Could you check a few things on this model? Use its own coordinates, in mm. Face numbers are marked on the shaded views. A direction names the side the tool comes from. Give positions to 0.01 mm unless a question says otherwise; leave off trailing zeros. Loops run counter-clockwise (first coordinate to the right, second up) from the corner with the lowest first, then second, coordinate; pieces in that order, holes last. Notation, with made-up numbers: (84.5, 22.25) - (94.5, 22.25) arc R24 cw to (94.5, 52.25) - close; hole circle Ø8 at (-19.5, 61.5). An arc over 180 degrees is marked (long way). One line per item, written item: value. Start each with the question number.
Q1. If I drill on line 1 (Z direction, x = -14, y = -12); line 2 (Y direction, x = -11, z = 5.5) (3 decimals); line 3 (Y direction, x = -13.5, z = 6.5), over which ranges is the centre line in solid material (lowest first)? Write a range as from..to.
Q2. I want a section at B-B (z = 2.75). Please give me the cut outline in (x, y), then the cut area to 3 significant figures.
Q3. I'm going to push flat-ended pins straight in: P1, Ø5, axis at y = 15, z = 13, coming from the +X side; P2, Ø2, axis at y = 40, z = 17.5, coming from the +X side; P3, Ø2.5, axis at x = 20, y = 0, coming from the +Z side; P4, Ø4.5, axis at x = -20, y = 0, coming from the +Z side. Where does each tip first touch, or does it pass through?
Q4. If we mould it in two halves opening along Y, with no side actions, what happens to the marked faces 5, 6 and 7? For each: released by +Y, released by -Y, zero draft, split by the parting line, or undercut.
Q5. I want a section at C-C (x = -20). Please give me the cut outline in (y, z), then the cut area to 3 significant figures.
Q6. For the marked faces 1, 2, 3 and 4, which set-ups out of +Z, -Z, +X, -X, +Y, -Y let a thin tool reach every point of the face, with its end or its side?
Q7. I want a section at D-D (y = -7). Please give me the cut outline in (x, z), then the cut area to 3 significant figures.
Q8. I want a section at A-A (z = 13). Count the separate pieces of the cut face and the enclosed holes in it, then the cut area to 3 significant figures.
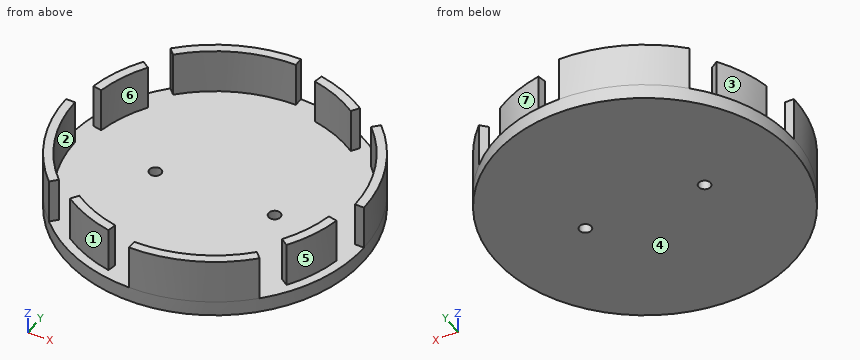
```python
from build123d import *
from build123d.topology import SkipClean

# Parameters (mm, degrees)
SKETCH_1_R      = 50
SKETCH_1_R_2    = 2
EXTRUDE_1_DEPTH = 5
EXTRUDE_2_DEPTH = 15
EXTRUDE_3_DEPTH = 15
EXTRUDE_4_DEPTH = 15


with BuildPart() as part:
    # 草图1 → 凸台-拉伸1 (new body)
    with BuildSketch(Plane.XY):
        Circle(SKETCH_1_R)
        with Locations((-20, 0)):
            Circle(SKETCH_1_R_2, mode=Mode.SUBTRACT)
        with Locations((20, 0)):
            Circle(SKETCH_1_R_2, mode=Mode.SUBTRACT)
    extrude(amount=EXTRUDE_1_DEPTH)

    # 草图2 → 凸台-拉伸2 (add)
    with SkipClean():  # the faces are left unmerged after this step: merging them gives an invalid solid
        with BuildSketch(Plane.XY.offset(5)):
            with BuildLine():
                Line((0, 50), (0, 47))
                ThreePointArc((0, 47), (-17.986121321, 43.422338028), (-33.234018716, 33.234018716))
                Line((-33.234018716, 33.234018716), (-35.355339059, 35.355339059))
                ThreePointArc((-35.355339059, 35.355339059), (-19.134171618, 46.193976626), (0, 50))
            make_face()
        extrude(amount=EXTRUDE_2_DEPTH)

    # 草图5 → 凸台-拉伸3 (add)
    with SkipClean():  # the faces are left unmerged after this step: merging them gives an invalid solid
        with BuildSketch(Plane.XY.offset(5)):
            with BuildLine():
                Line((-35.355339059, 35.355339059), (-33.234018716, 33.234018716))
                ThreePointArc((-33.234018716, 33.234018716), (-17.986121321, 43.422338028), (0, 47))
                Line((0, 47), (0, 50))
                ThreePointArc((0, 50), (-19.134171618, 46.193976626), (-35.355339059, 35.355339059))
            make_face()
            with BuildLine():
                Line((-50, 0), (-47, 0))
                ThreePointArc((-47, 0), (-43.422338028, -17.986121321), (-33.234018716, -33.234018716))
                Line((-33.234018716, -33.234018716), (-35.355339059, -35.355339059))
                ThreePointArc((-35.355339059, -35.355339059), (-46.193976626, -19.134171618), (-50, 0))
            make_face()
            with BuildLine():
                Line((33.234018716, 33.234018716), (35.355339059, 35.355339059))
                ThreePointArc((35.355339059, 35.355339059), (46.193976626, 19.134171618), (50, 0))
                Line((50, 0), (47, 0))
                ThreePointArc((47, 0), (43.422338028, 17.986121321), (33.234018716, 33.234018716))
            make_face()
            with BuildLine():
                Line((0, -47), (0, -50))
                ThreePointArc((0, -50), (19.134171618, -46.193976626), (35.355339059, -35.355339059))
                Line((35.355339059, -35.355339059), (33.234018716, -33.234018716))
                ThreePointArc((33.234018716, -33.234018716), (17.986121321, -43.422338028), (0, -47))
            make_face()
        extrude(amount=EXTRUDE_3_DEPTH)

    # 草图6 → 凸台-拉伸4 (add)
    with SkipClean():  # the faces are left unmerged after this step: merging them gives an invalid solid
        with BuildSketch(Plane.XY.offset(5)):
            with BuildLine():
                Line((-39.079071778, 26.111800952), (-36.584662941, 24.445090253))
                ThreePointArc((-36.584662941, 24.445090253), (-40.65069943, 16.838071024), (-43.154552338, 8.583974169))
                Line((-43.154552338, 8.583974169), (-46.096908179, 9.169245135))
                ThreePointArc((-46.096908179, 9.169245135), (-43.422338028, 17.986121321), (-39.079071778, 26.111800952))
            make_face()
            with BuildLine():
                Line((9.169245135, 46.096908179), (8.583974169, 43.154552338))
                ThreePointArc((8.583974169, 43.154552338), (16.838071024, 40.65069943), (24.445090253, 36.584662941))
                Line((24.445090253, 36.584662941), (26.111800952, 39.079071778))
                ThreePointArc((26.111800952, 39.079071778), (17.986121321, 43.422338028), (9.169245135, 46.096908179))
            make_face()
            with BuildLine():
                Line((46.096908179, -9.169245135), (43.154552338, -8.583974169))
                ThreePointArc((43.154552338, -8.583974169), (40.65069943, -16.838071024), (36.584662941, -24.445090253))
                Line((36.584662941, -24.445090253), (39.079071778, -26.111800952))
                ThreePointArc((39.079071778, -26.111800952), (43.422338028, -17.986121321), (46.096908179, -9.169245135))
            make_face()
            with BuildLine():
                Line((-9.169245135, -46.096908179), (-8.583974169, -43.154552338))
                ThreePointArc((-8.583974169, -43.154552338), (-16.838071024, -40.65069943), (-24.445090253, -36.584662941))
                Line((-24.445090253, -36.584662941), (-26.111800952, -39.079071778))
                ThreePointArc((-26.111800952, -39.079071778), (-17.986121321, -43.422338028), (-9.169245135, -46.096908179))
            make_face()
        extrude(amount=EXTRUDE_4_DEPTH)


solid = part.part
```
Worked answers:
1. line 1: z = 0..5
1. line 2: y = -45.695..-42.603, 45.695..48.775
1. line 3: y = -45.02..-41.88, 45.02..48.14
2. outline: circle Ø100 at (0, 0); hole circle Ø4 at (-20, 0); hole circle Ø4 at (20, 0)
2. area: 7,830 mm²
3. P1: stops at x = 48.41
3. P2: stops at x = 26.11
3. P3: passes through
3. P4: stops at z = 5
4. face 5: released by -Y
4. face 6: undercut
4. face 7: released by +Y
5. outline: (-45.83, 0) - (-2, 0) - (-2, 5) - (-39.19, 5) - (-39.19, 20) - (-42.53, 20) - (-42.53, 5) - (-45.83, 5) - close; (2, 0) - (45.83, 0) - (45.83, 20) - (42.53, 20) - (42.53, 5) - (2, 5) - close
5. area: 538 mm²
6. face 1: +Z, -X, -Y
6. face 2: +Z
6. face 3: +Z, -X, +Y
6. face 4: -Z, +X, -X, +Y, -Y
7. outline: (-49.51, 0) - (49.51, 0) - (49.51, 5) - (-46.48, 5) - (-46.48, 20) - (-49.51, 20) - close
7. area: 541 mm²
8. separate pieces: 8
8. enclosed holes: 0
8. area: 672 mm²
